```python
from build123d import *

# Parameters (mm, degrees)
F0_W     = 8
F0_H     = 15
F0_W_2   = 10
F0_H_2   = 30
F0_R     = 17.5
F1_DEPTH = 15
F2_R     = 2


with BuildPart() as f1:
    # F0 (on Top) → F1 (new body)
    with BuildSketch(Plane.XY):
        Polygon((-21.3343975244, -12.5), (-21.3343975244, 12.5), (-176.3343975244, 12.5), (-176.3343975244, -12.5), (-166.3343975244, -12.5), (-156.3343975244, -12.5), (-148.3343975244, -12.5), (-138.3343975244, -12.5), (-124.3343975244, -12.5), align=None)
        with Locations((-152.3343975244, -20)):
            Rectangle(F0_W, F0_H)
        with Locations((-171.3343975244, -27.5)):
            Rectangle(F0_W_2, F0_H_2)
        Polygon((-131.424844265, -27.5), (-124.3343975244, -12.5), (-138.3343975244, -12.5), align=None)
        with BuildLine():
            ThreePointArc((-21.3343975244, -12.5), (46.3573445521, 0), (-21.3343975244, 12.5))
            Line((-21.3343975244, 12.5), (-21.3343975244, -12.5))
        make_face()
        with Locations((11.3573445521, 0)):
            Circle(F0_R, mode=Mode.SUBTRACT)
    extrude(amount=F1_DEPTH)

    # F2
    f2_edges = [f1.edges().sort_by_distance(p)[0] for p in [
        (-98.834398, 12.5, 15),
        (-72.834398, -12.5, 15),
        (-127.879621, -20, 15),
        (-134.879621, -20, 15),
        (-148.334398, -20, 15),
        (-143.334398, -12.5, 15),
        (-161.334398, -12.5, 15),
        (-166.334398, -27.5, 15),
        (-171.334398, -42.5, 15),
        (-176.334398, -15, 15),
        (46.357345, 0, 15),
        (-6.142655, 0, 15),
        (-98.834398, 12.5, 0),
        (-72.834398, -12.5, 0),
        (-127.879621, -20, 0),
        (-143.334398, -12.5, 0),
        (-134.879621, -20, 0),
        (-148.334398, -20, 0),
        (46.357345, 0, 0),
        (-6.142655, 0, 0),
        (-176.334398, -15, 0),
        (-166.334398, -27.5, 0),
        (-161.334398, -12.5, 0),
    ]]
    fillet(f2_edges, radius=F2_R)


solid = f1.part
```
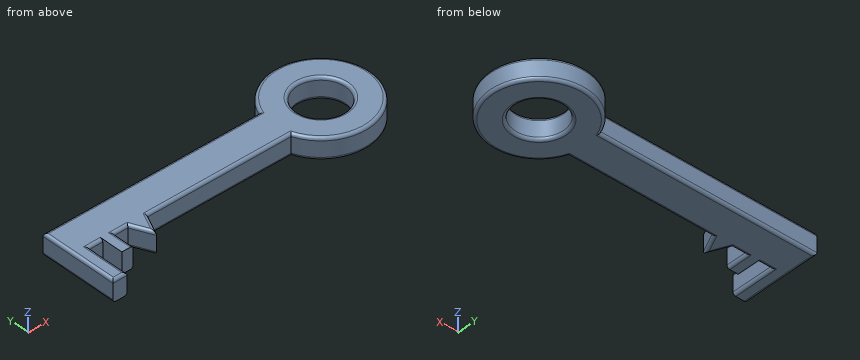
Geometry check sheet. Reference: the model listing, model coordinates, mm. Round coordinates to 2 decimals unless told otherwise and drop trailing zeros. Loops run counter-clockwise (first coordinate to the right, second up) from the corner with the lowest first, then second, coordinate; pieces in that order, holes last. Notation, with made-up numbers: (2, -38.5) - (9, -38.5) arc R31 cw to (9, -10.5) - close; hole circle Ø3 at (-39, -35.5). An arc over 180 degrees is marked (long way). Write each question's results on one line, items separated by ' | '. Start each with the question number.
Q1. Gauge pin test, flat ends, axial feed: P1, Ø1.5, axis at x = -92, y = 12.5, coming from the +Z side; P2, Ø3.5, axis at y = -33.5, z = 5.5, coming from the +X side; P3, Ø5, axis at y = -15, z = 4.5, coming from the +X side. Record the tip position at first contact, or that the pin passes through.
Q2. Cross-section at A-A on z = 10. Enter the section's corners in (x, y).
Q3. Cross-section at B-B on x = -100.5. Enter the section's corners in (y, z), and give its area (3 significant figures).
Q4. Thickness scan on line 1 (X direction, y = -21, z = 12.75); line 2 (X direction, y = -22, z = 3); line 3 (Y direction, x = -23.5, z = 11.25). Record the ranges inside material, lowest first. Write a range as [from, to].
Answers below:
1) P1: stops at z = 14.56 | P2: stops at x = 26.09 | P3: stops at x = 44.05
2) outline: (-176.33, -42.5) - (-166.33, -42.5) - (-166.33, -12.5) - (-156.33, -12.5) - (-156.33, -27.5) - (-148.33, -27.5) - (-148.33, -12.5) - (-138.33, -12.5) - (-131.42, -27.5) - (-124.33, -12.5) - (-21.33, -12.5) arc R35 ccw (long way) to (-21.33, 12.5) - (-176.33, 12.5) - close; hole circle Ø35 at (11.36, 0)
3) outline: (-12.5, 2) arc R2 ccw to (-10.5, 0) - (10.5, 0) arc R2 ccw to (12.5, 2) - (12.5, 13) arc R2 ccw to (10.5, 15) - (-10.5, 15) arc R2 ccw to (-12.5, 13) - close | area: 372 mm²
4) line 1: x = [-176.33, -166.33], [-156.33, -148.33], [-134.42, -128.35], [-16.64, 39.36] | line 2: x = [-176.33, -166.33], [-156.33, -148.33], [-133.96, -128.83], [-15.86, 38.58] | line 3: y = [-12.5, 12.5]
